Model file for the job. Use its own axes, mm. Face numbers are marked on the shaded views. Coordinates: 2 decimals unless noted, no trailing zeros. Write each loop counter-clockwise with the first axis right and the second up, starting at its lowest first coordinate (ties: lowest second). Pieces come first, ordered by that corner, then holes. Notation, with made-up numbers: (-15, 8.25) - (5, 8.25) arc R29 cw to (5, 44.25) - close; hole circle Ø3 at (39, 57.5). An arc over 180 degrees is marked (long way). Put each result on its own line as item: value. Start each with the question number.
1. Saw through at A-A, the plane x = 0. Write the cut outline in (y, z), plus the area to 3 significant figures.
2. Drill centre lines: L1, parallel to Z at x = 0, y = -10; L2, parallel to Y at x = 0, z = -5.5; L3, parallel to X at y = -6.5, z = 3.25. Where is each one in solid material? Low to high. Write a range as from..to.
3. Saw through at B-B, the plane y = -5.25. Write the cut outline in (x, z).
4. Pull direction X, two halves, no side cores. Call the marked faces 1, 2 and 3: released by +X, released by -X, zero draft, split by the parting line, or undercut.
5. Drop flat-ended pins along their axis: P1, Ø6.5, axis at x = -3, z = 3, coming from the -Y side; P2, Ø1, axis at x = 1, y = -1.5, coming from the +Z side; P3, Ø3, axis at x = -6.5, y = -2, coming from the -Z side (3 decimals); P4, Ø1.5, axis at x = -4, y = -7.5, coming from the -Z side. Give the stop position or say it passes through.
6. Saw through at C-C, the plane y = -1.5. Write the cut outline in (x, z), plus the area to 3 significant figures.
```python
from build123d import *

# Parameters (mm, degrees)
F0_R     = 8
F0_R_2   = 6.5
F1_DEPTH = 12
F2_R     = 1
F3_R     = 7
F3_R_2   = 6.5
F4_DEPTH = 2


with BuildPart() as f1:
    # F0 (on Front) → F1 (new body)
    with BuildSketch(Plane.XZ):
        Circle(F0_R)
        Circle(F0_R_2, mode=Mode.SUBTRACT)
    extrude(amount=F1_DEPTH)

    # F2
    f2_edges = [f1.edges().sort_by_distance(p)[0] for p in [
        (-8, -12, 0),
        (-8, 0, 0),
    ]]
    fillet(f2_edges, radius=F2_R)

    # F3 (on face) → F4 (join)
    with BuildSketch(Plane(origin=(0, 0, 0), x_dir=(-1, 0, 0), z_dir=(0, 1, 0))):
        Circle(F3_R)
        Circle(F3_R_2, mode=Mode.SUBTRACT)
        Circle(F3_R_2)
    extrude(amount=-F4_DEPTH)


solid = f1.part
```
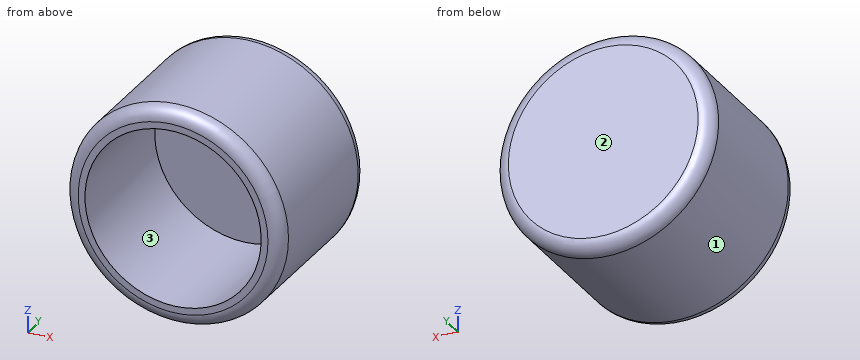
Final values:
1. outline: (-12, -7) arc R1 ccw to (-11, -8) - (-1, -8) arc R1 ccw to (0, -7) - (0, 7) arc R1 ccw to (-1, 8) - (-11, 8) arc R1 ccw to (-12, 7) - (-12, 6.5) - (-2, 6.5) - (-2, -6.5) - (-12, -6.5) - close
1. area: 61.1 mm²
2. L1: z = -8..-6.5, 6.5..8
2. L2: y = -2..0
2. L3: x = -7.31..-5.63, 5.63..7.31
3. outline: circle Ø16 at (0, 0); hole circle Ø13 at (0, 0)
4. face 1: split by the parting line
4. face 2: zero draft
4. face 3: undercut
5. P1: stops at y = -12
5. P2: stops at z = 7.98
5. P3: stops at z = -6.245
5. P4: stops at z = -7.31
6. outline: circle Ø16 at (0, 0)
6. area: 201 mm²
